from build123d import *

# Parameters (mm, degrees)
F0_R     = 4.5
F1_DEPTH = 27
F2_DEPTH = 2


with BuildPart() as f1:
    # F0 (on Top) → F1 (new body)
    with BuildSketch(Plane.XY):
        with BuildLine():
            ThreePointArc((-29.591673, -1), (-29.522966, -0.502097), (-29.5, 0))
            ThreePointArc((-29.5, 0), (-29.522966, 0.502097), (-29.591673, 1))
            ThreePointArc((-29.591673, 1), (-40.5, 0), (-29.591673, -1))
        make_face()
        with Locations((-35, 0)):
            Circle(F0_R, mode=Mode.SUBTRACT)
    extrude(amount=F1_DEPTH)

    # F0 (on Top) → F2 (join)
    with BuildSketch(Plane.XY):
        with BuildLine():
            ThreePointArc((-29.591673, 1), (-29.522966, 0.502097), (-29.5, 0))
            ThreePointArc((-29.5, 0), (-29.522966, -0.502097), (-29.591673, -1))
            Line((-29.591673, -1), (0, -1))
            Line((0, -1), (0, 1))
            Line((0, 1), (-29.591673, 1))
        make_face()
    extrude(amount=F2_DEPTH)

    # F3: F1 across plane


with BuildPart() as f1_1:
    add(f1.part)
    add(f1.part.mirror(Plane.YZ))


solid = f1_1.part
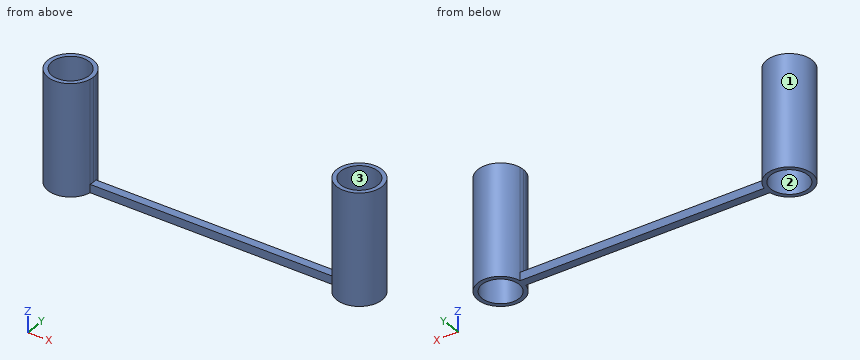
The listing builds one solid part. Answer for the finished solid, in the listing's coordinates (mm). Face numbers are marked on the shaded views. Give positions to 0.01 mm unless a question says otherwise; leave off trailing zeros. Order: outer loops, then holes, each group sorted by start corner. A loop starts at its lowest first (then second) coordinate and runs counter-clockwise, first axis right, second up. Notation, with made-up numbers: (59.5, 42.25) - (91.5, 42.25) arc R34 cw to (91.5, 76.25) - close; hole circle Ø1 at (-10, 12.5). An arc over 180 degrees is marked (long way). One line per item, written item: value. Start each with the question number.
1) Find the intervals of material crossed by L1, parallel to X at y = 3.25, z = 18.75; L2, parallel to Y at x = 35, z = 14; L3, parallel to X at y = 2.5, z = 12.5, in increasing order.
2) A cutting plane is placed at D-D on x = 26. Give the vertices of the cut face in (y, z), then the cut area to 3 significant figures.
3) A cutting plane is placed at A-A on z = 16.5. Give the vertices of the cut face in (x, y), then the cut area to 3 significant figures.
4) A cutting plane is placed at B-B on x = -35. Give the vertices of the cut face in (y, z).
5) The mould has two halves that part along Y. Classify the marked faces 1, 2 and 3: released by +Y, released by -Y, zero draft, split by the parting line, or undercut.
6) A cutting plane is placed at C-C on y = 3. Give the vertices of the cut face in (x, z), then the cut area to 3 significant figures.
7) Given pin 1 Ø0.6 at (x, z) = (-1.5, 1.5) entering from -Y; pin 2 Ø5 at (y, z) = (3.5, 7) entering from -X; pin 3 Ø1 at (x, y) = (-5.5, 0.5) entering from +Z; pin 4 Ø3 at (x, y) = (-28.5, -4) entering from -Z, each flat-ended and moving along its own axis, determine where each tip first touches the part or whether it passes through.
Answer sheet:
1. L1: x = -39.44 to -38.11, -31.89 to -30.56, 30.56 to 31.89, 38.11 to 39.44
1. L2: y = -5.5 to -4.5, 4.5 to 5.5
1. L3: x = -39.9 to -38.74, -31.26 to -30.1, 30.1 to 31.26, 38.74 to 39.9
2. outline: (-1, 0) - (1, 0) - (1, 2) - (-1, 2) - close
2. area: 4.00 mm2
3. outline: (-29.59, -1) arc R5.5 ccw to (-29.5, 0) arc R5.5 ccw to (-29.59, 1) arc R5.5 ccw (long way) to start; (29.5, 0) arc R5.5 ccw to (29.59, -1) arc R5.5 ccw (long way) to (29.59, 1) arc R5.5 ccw to start; hole circle Ø9 at (-35, 0); hole circle Ø9 at (35, 0)
3. area: 62.8 mm2
4. outline: (-5.5, 0) - (-4.5, 0) - (-4.5, 27) - (-5.5, 27) - close; (4.5, 0) - (5.5, 0) - (5.5, 27) - (4.5, 27) - close
5. face 1: split by the parting line
5. face 2: undercut
5. face 3: undercut
6. outline: (-39.61, 0) - (-38.35, 0) - (-38.35, 27) - (-39.61, 27) - close; (-31.65, 0) - (-30.39, 0) - (-30.39, 27) - (-31.65, 27) - close; (30.39, 0) - (31.65, 0) - (31.65, 27) - (30.39, 27) - close; (38.35, 0) - (39.61, 0) - (39.61, 27) - (38.35, 27) - close
6. area: 136 mm2
7. pin 1: stops at y = -1
7. pin 2: stops at x = -40.41
7. pin 3: stops at z = 2
7. pin 4: passes through
